Work out the finished part from the listing and answer in its coordinate system (mm). Face numbers are marked on the shaded views. A direction names the side the tool comes from. Coordinates: 2 decimals unless noted, no trailing zeros. Order: outer loops, then holes, each group sorted by start corner. A loop starts at its lowest first (then second) coordinate and runs counter-clockwise, first axis right, second up. Notation, with made-up numbers: M 55.5,30.5 L 76.5,30.5 A28 cw 76.5,62.5 Z; hole C -12,-34.75 d11. An arc over 180 degrees is marked long. Use a Markdown table: item, result. Add a question column.
from build123d import *

# Parameters (mm, degrees)
F0_R      = 19
F1_DEPTH  = 57.1
F2_R      = 16
F3_DEPTH  = 41.8
F4_R      = 16
F5_DEPTH  = 10
F7_DEPTH  = 3
F8_R      = 3
F9_DEPTH  = 16.2
F10_W     = 3.3166247904
F10_H     = 0.5
F11_DEPTH = 12
F12_SIZE  = 2
F14_D     = 2.5
F14_DEPTH = 13.5
F14_TIP   = 0.7510757738


with BuildPart() as f1:
    # F0 (on Top) → F1 (new body)
    with BuildSketch(Plane.XY):
        Circle(F0_R)
    extrude(amount=-F1_DEPTH)

    # F2 (on face) → F3 (join)
    with BuildSketch(Plane.XY):
        Circle(F2_R)
    extrude(amount=F3_DEPTH)

    # F4 (on face) → F5 (join)
    with BuildSketch(Plane(origin=(0, 0, -57.1), x_dir=(1, 0, 0), z_dir=(0, 0, -1))):
        Circle(F4_R)
    extrude(amount=F5_DEPTH)

    # F6 (on face) → F7 (join)
    with BuildSketch(Plane.XY.offset(41.8)):
        with BuildLine():
            ThreePointArc((9, 4.3588989435), (0, 10), (-9, 4.3588989435))
            Line((-9, 4.3588989435), (-9, -4.3588989435))
            ThreePointArc((-9, -4.3588989435), (0, -10), (9, -4.3588989435))
            Line((9, -4.3588989435), (9, 4.3588989435))
        make_face()
    extrude(amount=F7_DEPTH)

    # F8 (on face) → F9 (join)
    with BuildSketch(Plane.XY.offset(44.8)):
        Circle(F8_R)
    extrude(amount=F9_DEPTH)

    # F10 (on face) → F11 (cut)
    with BuildSketch(Plane.XY.offset(61)):
        with Locations((0, 2.75)):
            Rectangle(F10_W, F10_H)
    extrude(amount=-F11_DEPTH, mode=Mode.SUBTRACT)

    # F12
    f12_edges = [f1.edges().sort_by_distance(p)[0] for p in [
        (-19, 0, -57.1),
        (-19, 0, 0),
    ]]
    chamfer(f12_edges, length=F12_SIZE)

    # F14
    with Locations(Plane.XY.offset(41.8)):
        with Locations((-9.1923881554, 9.1923881554), (9.1923881554, 9.1923881554), (9.1923881554, -9.1923881554), (-9.1923881554, -9.1923881554)):
            Hole(F14_D / 2, depth=F14_DEPTH)
            with Locations((0, 0, -(F14_DEPTH + F14_TIP / 2))):  # 118° drill point
                Cone(0, F14_D / 2, F14_TIP, mode=Mode.SUBTRACT)


solid = f1.part
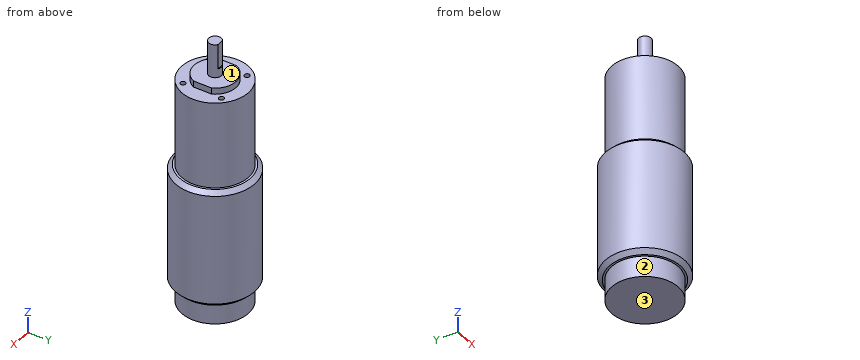
(1) Straight lines are drawn through the part: line 1 (Z direction, x = 4, y = -12); line 2 (Y direction, x = 0, z = -23); line 3 (Z direction, x = 5, y = 0). For each, find the intervals that lie inside material, in ascending order.
(2) Given P1, Ø0.9, axis at y = -1, z = 43, coming from the -X side; P2, Ø3, axis at y = 8, z = 46, coming from the -X side; P3, Ø4, axis at x = 14.5, z = -14.5, coming from the -Y side, each flat-ended and moving along its own axis, determine where each tip first touches the part or whether it passes through.
(3) A cutting plane is placed at D-D on z = 51.5. Write down the section's boundary in (x, y).
(4) A cutting plane is placed at B-B on x = 0. Write down the section's boundary in (y, z), plus the area to 3 significant figures.
(5) A cutting plane is placed at C-C on z = -16.5. Write down the section's boundary in (x, y).
(6) Which of the six approach directions +Z, -Z, +X, -X, +Y, -Y give full straight-line access (tool end or side, diameter ignored) to the marked faces 1, 2 and 3?
(7) A cutting plane is placed at A-A on y = 0. Write down the section's boundary in (x, z).
From the geometry:
| question | item | result |
|---|---|---|
| 1 | line 1 | z = -67.1 to 41.8 |
| 1 | line 2 | y = -19 to 19 |
| 1 | line 3 | z = -67.1 to 44.8 |
| 2 | P1 | stops at x = -9 |
| 2 | P2 | stops at x = -7.04 |
| 2 | P3 | stops at y = -14.31 |
| 3 | outline | M -1.66,2.5 A3 ccw long 1.66,2.5 Z |
| 4 | outline | M -19,-55.1 L -17,-57.1 L -16,-57.1 L -16,-67.1 L 16,-67.1 L 16,-57.1 L 17,-57.1 L 19,-55.1 L 19,-2 L 17,0 L 16,0 L 16,41.8 L 10,41.8 L 10,44.8 L 3,44.8 L 3,49 L 2.5,49 L 2.5,61 L -3,61 L -3,44.8 L -10,44.8 L -10,41.8 L -16,41.8 L -16,0 L -17,0 L -19,-2 Z |
| 4 | area | 3,970 mm2 |
| 5 | outline | C 0,0 d38 |
| 6 | face 1 | +Z |
| 6 | face 2 | -Z |
| 6 | face 3 | -Z, +X, -X, +Y, -Y |
| 7 | outline | M -19,-55.1 L -17,-57.1 L -16,-57.1 L -16,-67.1 L 16,-67.1 L 16,-57.1 L 17,-57.1 L 19,-55.1 L 19,-2 L 17,0 L 16,0 L 16,41.8 L 9,41.8 L 9,44.8 L 3,44.8 L 3,61 L -3,61 L -3,44.8 L -9,44.8 L -9,41.8 L -16,41.8 L -16,0 L -17,0 L -19,-2 Z |
